```python
from build123d import *

# Parameters (mm, degrees)
BOSS_EXTRUDE1_DEPTH = 4.064
SKETCH2_R           = 0.762
CUT_EXTRUDE1_DEPTH  = 5.996401933


with BuildPart() as part:
    # Sketch1 → Boss-Extrude1 (new body)
    with BuildSketch(Plane(origin=(0, 0, 0), x_dir=(0, 0, -1), z_dir=(1, 0, 0))):
        with BuildLine():
            Line((4.726865031, 5.556764983), (4.726865031, -0.444820699))
            ThreePointArc((4.726865031, -0.444820699), (2.554182799, -2.454658405), (-0.22039607, -3.485050462))
            ThreePointArc((-0.22039607, -3.485050462), (-4.22007249, -7.510942511), (-1.625042246, -12.557826332))
            Line((-1.625042246, -12.557826332), (-1.435472167, -12.557826332))
            add(Edge.make_bspline(
                [(-1.435472167, -12.557826332), (-1.175924208, -12.557849399), (-0.648911083, -12.519392405), (0.32614537, -12.308921718), (1.440239513, -11.841665003), (2.626862444, -11.096563597), (4.080334858, -10.011065793), (5.769221033, -8.746934213), (7.066078237, -8.323424357), (7.761067398, -8.323424519)],
                knots=[0, 0, 0, 0, 0.054765757, 0.109531513, 0.219063026, 0.328594539, 0.438126053, 0.657189079, 0.876252105, 0.876252105, 0.876252105, 0.876252105], degree=3))
            Line((7.761067398, -8.323424519), (13.22812784, -8.323424519))
            Line((13.22812784, -8.323424519), (13.22812784, -7.561424519))
            Line((13.22812784, -7.561424519), (7.761067576, -7.561424519))
            add(Edge.make_bspline(
                [(-1.435404445, -11.795826335), (1.654785659, -11.796100971), (4.006866827, -8.222316999), (7.226557461, -7.561424394), (7.761067576, -7.561424519)],
                knots=[0, 0, 0, 0, 0.739499728, 0.876252105, 0.876252105, 0.876252105, 0.876252105], degree=3))
            ThreePointArc((-1.435404445, -11.795826335), (-3.452810626, -7.541681499), (-0.098895233, -4.237301448))
            ThreePointArc((-0.098895233, -4.237301448), (3.060460139, -3.036798555), (5.488865031, -0.686142637))
            Line((5.488865031, -0.686142637), (5.488865031, 5.556764983))
            Line((5.488865031, 5.556764983), (4.726865031, 5.556764983))
        make_face()
    extrude(amount=-BOSS_EXTRUDE1_DEPTH)

    # Sketch2 → Cut-Extrude1 (cut, through all)
    with BuildSketch(Plane(origin=(0, -7.561424519, 0), x_dir=(1, 0, 0), z_dir=(0, 1, 0))):
        with Locations((-2.032, 11.45012784)):
            Circle(SKETCH2_R)
    extrude(amount=-CUT_EXTRUDE1_DEPTH, mode=Mode.SUBTRACT)


solid = part.part
```
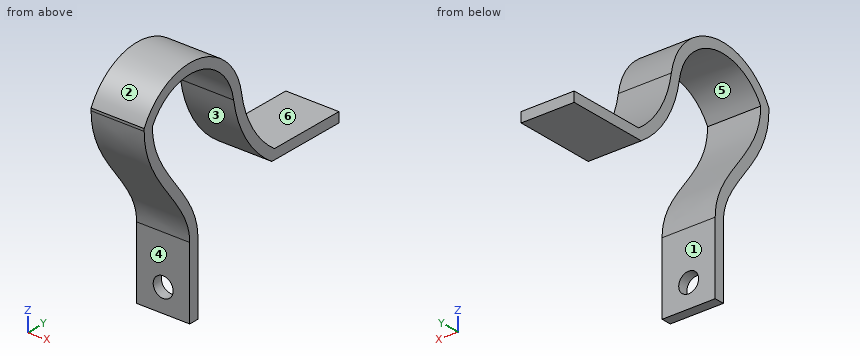
Check sheet for the modelled part. Datum: model origin and axes. Units: mm. Face numbers are marked on the shaded views. A direction names the side the tool comes from. Give positions to 0.01 mm unless a question says otherwise; leave off trailing zeros. Order: outer loops, then holes, each group sorted by start corner. A loop starts at its lowest first (then second) coordinate and runs counter-clockwise, first axis right, second up. Notation, with made-up numbers: (-17, -24.5) -> (37, -24.5) arc R35 cw to (37, 14.5) -> close; hole circle Ø7 at (-25.5, -7). An arc over 180 degrees is marked (long way). Use CSV: the item, a comma, the result in double quotes. Start each with the question number.
1) Mould release check, pull along Y, two halves, no side actions. Record for the marked faces 3, 4, 5 and 6: released by +Y, released by -Y, zero draft, split by the parting line, or undercut.
2) Sectioned sample at C-C, the plane y = -2. Record the boundary of the cut face in (x, z), plus the area to 3 significant figures.
3) Material ranges on line 1 (Z direction, x = -0.85, y = 4.75); line 2 (Z direction, x = -1.95, y = -10); line 3 (Y direction, x = -1.45, z = 2.75), recorded low to high. Write a range as from..to.
4) Set-up check for the marked faces 1 and 2: record each of +Z, -Z, +X, -X, +Y, -Y from which the full face is reachable in a straight line by a thin tool's end or side.
5) Go/stop test with flat-tipped pins: P1, Ø2, axis at x = -2, z = -10.5, coming from the +Y side; P2, Ø2, axis at x = -2.5, z = -11, coming from the -Y side; P3, Ø2, axis at x = -3, y = 2.5, coming from the +Z side. Record where each tip stops, or that it passes through.
6) Sectioned sample at A-A, the plane z = -12. Record the boundary of the cut face in (x, y).
7) Sectioned sample at B-B, the plane z = -10. Record the boundary of the cut face in (x, y), plus the area to 3 significant figures.
Recorded:
1,face 3,"undercut"
1,face 4,"released by -Y"
1,face 5,"undercut"
1,face 6,"zero draft"
2,outline,"(-4.06, -4.38) -> (0, -4.38) -> (0, -3.21) -> (-4.06, -3.21) -> close"
2,area,"4.74 mm2"
3,line 1,"-5.49..-4.73"
3,line 2,"-4.1..-2.82, 3.12..3.95"
3,line 3,"-11.77..-10.62, -5.88..-4.73"
4,face 1,"-Z, +X, -X, +Y"
4,face 2,"+Z, +X, -X"
5,P1,"y = -7.56"
5,P2,"y = -8.32"
5,P3,"z = -4.73"
6,outline,"(-4.06, -8.32) -> (-2.56, -8.32) -> (-2.56, -7.56) -> (-4.06, -7.56) -> close; (-1.5, -8.32) -> (0, -8.32) -> (0, -7.56) -> (-1.5, -7.56) -> close"
7,outline,"(-4.06, -8.32) -> (0, -8.32) -> (0, -7.56) -> (-4.06, -7.56) -> close"
7,area,"3.10 mm2"
